Could you check a few things on this drawing? It's one solid part, dimensions in mm from its lowest x, y, z. A direction names the side the tool comes from. Round coordinates to 2 decimals unless told otherwise and drop trailing zeros. Write each loop counter-clockwise with the first axis right and the second up, starting at its lowest first coordinate (ties: lowest second). Pieces come first, ordered by that corner, then holes. Notation, with made-up numbers: M 47,84 L 73,84 A28 ccw 73,110 Z; hole C 44,30.5 d1. An arc over 180 degrees is marked long. One line per item, written item: value. Start each with the question number.
(1) I'm going to push flat-ended pins straight in: pin 1 Ø5.5 at (x, z) = (48.6, 7) entering from -Y; pin 2 Ø4.5 at (x, z) = (5, 7) entering from +Y; pin 3 Ø3 at (x, z) = (5, 40) entering from -Y; pin 4 Ø1 at (x, z) = (28.5, 29.5) entering from +Y. Where does each tip first touch, or does it pass through?
(2) I want a section at C-C on z = 7. Please give me the cut outline in (x, y), and give its area (3 significant figures).
(3) Which directions (+Z, -Z, +X, -X, +Y, -Y) give clear straight access to the entire face, cutting with the end or side of a thin tool? Please do the marked faces 1, 2 and 3.
(4) Thinking about a two-plate mould opening in X: for the marked faces 4, 5 and 6, which applies, released by +X, released by -X, zero draft, split by the parting line, or undercut?
(5) I want a section at D-D on z = 37.5. Please give me the cut outline in (x, y).
(6) I want a section at B-B on y = 11. Please give me the cut outline in (x, z).
(7) I want a section at A-A on x = 5. Please give me the cut outline in (y, z), and give its area (3 significant figures).
(8) If I drill on L1, parallel to Z at x = 5, y = 1.25; L2, parallel to Y at x = 26.5, z = 18.5; L3, parallel to X at y = 3.5, z = 7.5, over which ranges is the centre line in solid material (lowest first)?
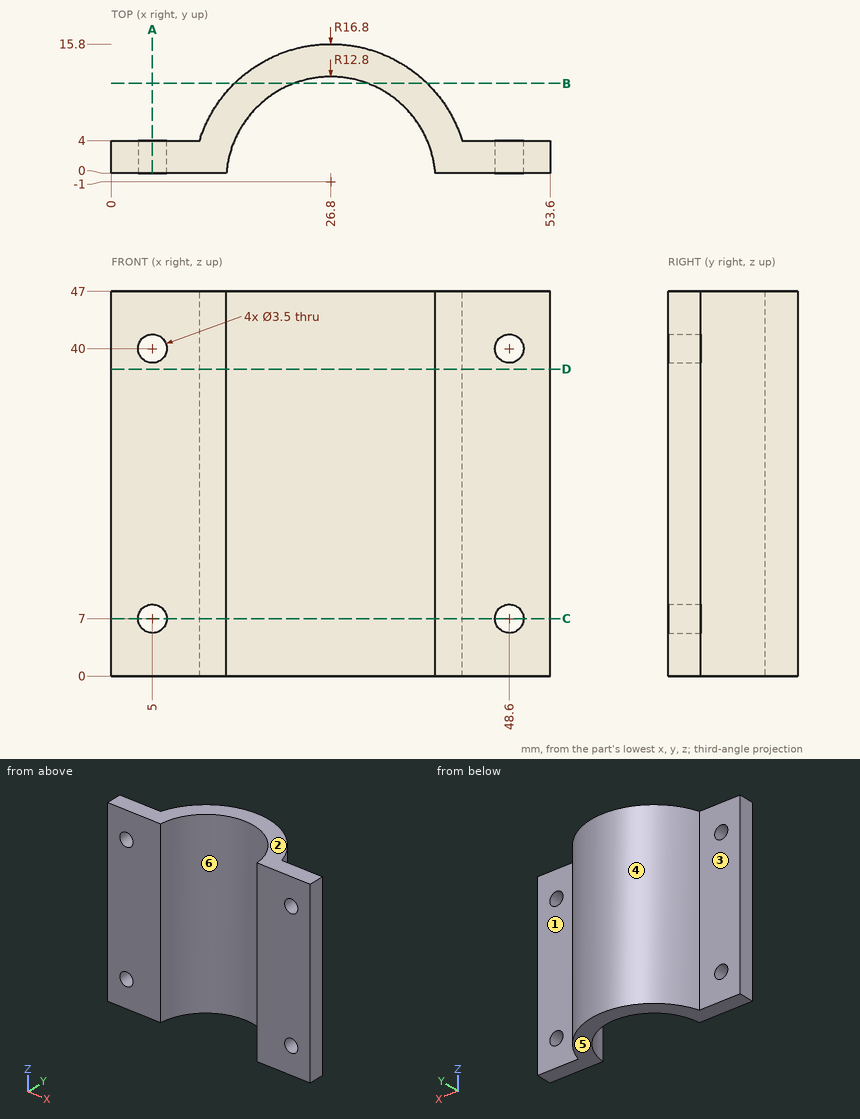
Found:
1. pin 1: stops at y = 0
1. pin 2: stops at y = 4
1. pin 3: passes through
1. pin 4: stops at y = 15.76
2. outline: M 0,0 L 3.25,0 L 3.25,4 L 0,4 Z; M 6.75,0 L 14.04,0 A12.8 cw 39.56,0 L 46.85,0 L 46.85,4 L 42.84,4 A16.8 ccw 10.76,4 L 6.75,4 Z; M 50.35,0 L 53.6,0 L 53.6,4 L 50.35,4 Z
2. area: 232 mm²
3. face 1: +Z, -Z, +X, +Y
3. face 2: +Z, +X, -X, +Y, -Y
3. face 3: +Z, -Z, -X, +Y
4. face 4: split by the parting line
4. face 5: zero draft
4. face 6: undercut
5. outline: M 0,0 L 14.04,0 A12.8 cw 39.56,0 L 53.6,0 L 53.6,4 L 42.84,4 A16.8 ccw 10.76,4 L 0,4 Z
6. outline: M 15.04,0 L 22.35,0 L 22.35,47 L 15.04,47 Z; M 31.25,0 L 38.56,0 L 38.56,47 L 31.25,47 Z
7. outline: M 0,0 L 4,0 L 4,5.25 L 0,5.25 Z; M 0,8.75 L 4,8.75 L 4,38.25 L 0,38.25 Z; M 0,41.75 L 4,41.75 L 4,47 L 0,47 Z
7. area: 160 mm²
8. L1: z = 0 to 5.25, 8.75 to 38.25, 41.75 to 47
8. L2: y = 11.8 to 15.8
8. L3: x = 0 to 3.32, 6.68 to 14.82, 38.78 to 46.92, 50.28 to 53.6
